from build123d import *

# Parameters (mm, degrees)
BASETOP_FACE_RADIUS = 4.02
BASETOP_HEIGHT      = 1
CROSSRECESS_DEPTH   = 1.35
DRAFT9_ANGLE        = -30
FILLET5_R           = 0.3


with BuildPart() as part:
    # Sketch1 → Base (revolve)
    with BuildSketch(Plane.XY, mode=Mode.PRIVATE) as base_sk:
        Polygon((16, 2), (4.187867966, 2), (2.408867966, 2), (0.388867966, 4.02), (0, 4.02), (0, 0), (16, 0), align=None)
    revolve(base_sk.sketch.rotate(Axis((4.515812911, 0, 0), (-1, 0, 0)), 90), axis=Axis((4.515812911, 0, 0), (-1, 0, 0)))

    # BaseTop: a dome of height H over a round flat face of radius A is a cap of a sphere of radius (A * A + H * H) / (2 * H)
    basetop_r = (BASETOP_FACE_RADIUS * BASETOP_FACE_RADIUS + BASETOP_HEIGHT * BASETOP_HEIGHT) / (2 * BASETOP_HEIGHT)
    basetop_base = Plane((0, 0, 0), z_dir=(-1, 0, 0))
    with Locations(basetop_base.offset(BASETOP_HEIGHT - basetop_r)):
        basetop_ball = Sphere(basetop_r, mode=Mode.PRIVATE)
    add(split(basetop_ball, bisect_by=basetop_base, keep=Keep.TOP, mode=Mode.PRIVATE))

    # Sketch6 → CrossRecess (cut)
    with BuildSketch(Plane.ZY.offset(1)):
        Polygon((0.52, 0.52), (0.52, 2.6), (-0.52, 2.6), (-0.52, 0.52), (-2.6, 0.52), (-2.6, -0.52), (-0.52, -0.52), (-0.52, -2.6), (0.52, -2.6), (0.52, -0.52), (2.6, -0.52), (2.6, 0.52), align=None)
    extrude(amount=-CROSSRECESS_DEPTH, mode=Mode.SUBTRACT)

    # Draft9
    draft9_faces = [part.faces().sort_by_distance(p)[0] for p in [
        (-0.120548575, 0, -2.6),
        (-0.120548575, -2.6, 0),
        (-0.120548575, 0, 2.6),
        (-0.120548575, 2.6, 0),
    ]]
    draft(draft9_faces, Plane(origin=(-1, 0, 0), x_dir=(0, 0, 1), z_dir=(1, 0, 0)), DRAFT9_ANGLE)

    # Fillet5
    fillet5_edges = [part.edges().sort_by_distance(p)[0] for p in [
        (-0.309213747, 0.52, -0.52),
        (-0.309213747, 0.52, 0.52),
        (-0.309213747, -0.52, 0.52),
        (-0.309213747, -0.52, -0.52),
    ]]
    fillet(fillet5_edges, radius=FILLET5_R)


solid = part.part
Design review of the part built by this model. Coordinates are the model's own, in mm. A direction names the side the tool comes from. Give positions to 0.01 mm unless a question says otherwise; leave off trailing zeros. Write each loop counter-clockwise with the first axis right and the second up, starting at its lowest first coordinate (ties: lowest second). Pieces come first, ordered by that corner, then holes. Notation, with made-up numbers: M -10.5,-0.75 L 34.5,-0.75 A9 ccw 34.5,6.25 Z; hole C 43.5,10 d10. An arc over 180 degrees is marked long. Return JSON: item names as keys, results as strings. Group by question number.
Item 1: Wall thickness on line 1 along X through (y, z) = (0, 0); line 2 along Y through (x, z) = (5, 0); line 3 along X through (y, z) = (2.5, 2): over which ranges is each line inside the solid? List them lowest first.
Item 2: The part is to be moulded in two halves that separate along Z. For faces 4 (the flat face through (0, -0.52, 1)), 5 (the flat face through (16, 0, 0)), 6 (the conical face through (2.28, 2.08, 0.46)), 7 (the flat face through (-0.161, 2.115, 0.007)), say which applies: pulls with the +Z half, pulls with the -Z half, needs draft (parallel to the pull), parting line crosses it, or undercut.
Item 3: Take a section at A-A (y = 0). Give the boundary of the cut face in (x, z), plus the area to 3 significant figures.
Item 4: Take a section at C-C (x = 6.25). Give the boundary of the cut face in (y, z).
Item 5: Tool access review of faces 1 (the cylindrical face through (0.192, -1.207, -3.834)), 2 (the flat face through (0, 1, 0.52)), 3 (the cylindrical face through (9, 2, 0)): name each direction out of +Z, -Z, +X, -X, +Y, -Y from which nothing blocks a thin tool from reaching the whole face with its end or side.
Item 6: Clearance check with flat-ended pins moving along their axes: pin 1 Ø1 at (x, y) = (0, -2) entering from -Z; pin 2 Ø1 at (x, z) = (0, -2) entering from -Y; pin 3 Ø1.4 at (x, z) = (-0.5, 1.5) entering from -Y. State where each tip first meets the part, or that it passes through.
Return value:
{
 "1": {"line 1": "x = 0.35 to 16", "line 2": "y = -2 to 2", "line 3": "x = -0.38 to 1.21"},
 "2": {"face 4": "undercut", "face 5": "needs draft", "face 6": "parting line crosses it", "face 7": "undercut"},
 "3": {"outline": "M -0.66,-2.4 A8.58 ccw 0,-4.02 L 0.39,-4.02 L 2.41,-2 L 16,-2 L 16,2 L 2.41,2 L 0.39,4.02 L 0,4.02 A8.58 ccw -0.66,2.4 L 0.35,1.82 L 0.35,-1.82 Z", "area": "69.7 mm2"},
 "4": {"outline": "C 0,0 d4"},
 "5": {"face 1": "+X, -X", "face 2": "-X", "face 3": "+X"},
 "6": {"pin 1": "stops at z = -3.73", "pin 2": "stops at y = -3.73", "pin 3": "stops at y = -3.89"}
}
